Can you work these out from the model? Positions are in its coordinate system, mm. Round coordinates to 2 decimals unless told otherwise and drop trailing zeros. Loops run counter-clockwise (first coordinate to the right, second up) from the corner with the lowest first, then second, coordinate; pieces in that order, holes last. Notation, with made-up numbers: (59.5, 73) - (97.5, 73) arc R22 cw to (97.5, 110) - close; hole circle Ø11 at (36.25, -12.75). An arc over 180 degrees is marked (long way). Answer as CSV lines item,"result".
```python
from build123d import *

# Parameters (mm, degrees)
BOSS_EXTRUDE1_DEPTH = 10
SKETCH2_R           = 2.5
CUT_EXTRUDE1_DEPTH  = 95.868329805
SKETCH4_R           = 2.5
CUT_EXTRUDE2_DEPTH  = 95.868329805
SKETCH5_R           = 2.5
CUT_EXTRUDE3_DEPTH  = 95.868329805


with BuildPart() as part:
    # Sketch1 → Boss-Extrude1 (new body)
    with BuildSketch(Plane(origin=(0, 0, 0), x_dir=(1, 0, 0), z_dir=(0, 1, 0))):
        with BuildLine():
            Line((-30, 50), (30, 50))
            ThreePointArc((30, 50), (37.071067812, 47.071067812), (40, 40))
            Line((40, 40), (40, -40))
            ThreePointArc((40, -40), (37.071067812, -47.071067812), (30, -50))
            Line((30, -50), (-30, -50))
            ThreePointArc((-30, -50), (-37.071067812, -47.071067812), (-40, -40))
            Line((-40, -40), (-40, 40))
            ThreePointArc((-40, 40), (-37.071067812, 47.071067812), (-30, 50))
        make_face()
    extrude(amount=BOSS_EXTRUDE1_DEPTH)

    # Sketch2 → Cut-Extrude1 (cut, through all)
    with BuildSketch(Plane(origin=(40, 0, 0), x_dir=(0, 0, -1), z_dir=(1, 0, 0))):
        with Locations((0, 4.743756571)):
            Circle(SKETCH2_R)
    extrude(amount=-CUT_EXTRUDE1_DEPTH, mode=Mode.SUBTRACT)

    # Sketch4 → Cut-Extrude2 (cut, through all)
    with BuildSketch(Plane(origin=(40, 0, 0), x_dir=(0, 0, -1), z_dir=(1, 0, 0))):
        with Locations((-28.371833373, 4.400978566)):
            Circle(SKETCH4_R)
    extrude(amount=-CUT_EXTRUDE2_DEPTH, mode=Mode.SUBTRACT)

    # Sketch5 → Cut-Extrude3 (cut, through all)
    with BuildSketch(Plane(origin=(40, 0, 0), x_dir=(0, 0, -1), z_dir=(1, 0, 0))):
        with Locations((28.154007397, 5.042029154)):
            Circle(SKETCH5_R)
    extrude(amount=-CUT_EXTRUDE3_DEPTH, mode=Mode.SUBTRACT)


solid = part.part
```
Q1. Imagine slicing it at C-C (x = 31.5). Write out the boundary of the cut face in (y, z), then the cut area to 3 significant figures.
Checks:
outline,"(0, -49.89) - (10, -49.89) - (10, 49.89) - (0, 49.89) - close; hole circle Ø5 at (4.4, 28.37); hole circle Ø5 at (4.74, 0); hole circle Ø5 at (5.04, -28.15)"
area,"939 mm²"
Q2. If I drill on line 1 along Y through (x, z) = (-3.5, 0); line 2 along Z through (x, y) = (-15, 5.25); line 3 along Z through (x, y) = (-12, 4.5), over which ranges is the centre line in solid material (lowest first)? Write a range as [from, to].
Checks:
line 1,"[0, 2.24], [7.24, 10]"
line 2,"[-50, -30.65], [-25.66, -2.45], [2.45, 26.02], [30.72, 50]"
line 3,"[-50, -30.59], [-25.71, -2.49], [2.49, 25.87], [30.87, 50]"
Q3. We'd pull the mould along Z, two halves only. Please class faces 1 (the flat face through (0, 5, 50)), 2 (the cylindrical face through (0.56, 4.08, -30.46)), 3 (the flat face through (1, 0, -1)), 4 (the cylindrical face through (36.99, 4.93, -47.15)): pulls with the +Z half, pulls with the -Z half, needs draft (parallel to the pull), parting line crosses it, or undercut.
Checks:
face 1,"pulls with the +Z half"
face 2,"undercut"
face 3,"needs draft"
face 4,"pulls with the -Z half"
Q4. Imagine slicing it at A-A (z = 0). Write out the boundary of the cut face in (x, y).
Checks:
outline,"(-40, 0) - (40, 0) - (40, 2.24) - (-40, 2.24) - close; (-40, 7.24) - (40, 7.24) - (40, 10) - (-40, 10) - close"
Q5. Imagine slicing it at B-B (x = -9). Write out the boundary of the cut face in (y, z), then the cut area to 3 significant figures.
Checks:
outline,"(0, -50) - (10, -50) - (10, 50) - (0, 50) - close; hole circle Ø5 at (4.4, 28.37); hole circle Ø5 at (4.74, 0); hole circle Ø5 at (5.04, -28.15)"
area,"941 mm²"
